Check sheet for the modelled part. Datum: model origin and axes. Units: mm. Round coordinates to 2 decimals unless told otherwise and drop trailing zeros. Loops run counter-clockwise (first coordinate to the right, second up) from the corner with the lowest first, then second, coordinate; pieces in that order, holes last. Notation, with made-up numbers: (-28, 86.25) -> (31, 86.25) arc R17 ccw to (31, 119.25) -> close; hole circle Ø4 at (1.5, 87). An arc over 180 degrees is marked (long way). Use one line per item in the form item = value. Start each with the question number.
(1) Draft check along Z on faces 1 (the cylindrical face through (29.32, 0.01, 86.79)), 2 (the cylindrical face through (-28.289, 0.011, 1.804)), 3 (the cylindrical face through (-24.263, 0.011, 5.805)). Enter one of: released by +Z, released by -Z, zero draft, split by the parting line, or undercut.
(2) Material ranges on probe 1 along X at (y, z) = (-0.2, 24); probe 2 along Z at (x, y) = (2.5, -0.65); probe 3 along X at (y, z) = (0.35, 83), recorded low to high. Write a range as [from, to].
(3) Sectioned sample at B-B (x = -25.75). Record the cut outline in (y, z).
(4) Sectioned sample at A-A (z = 24). Record the cut outline in (x, y), and give its area (3 significant figures).
(5) Go/stop test with flat-tipped pins: pin 1 (0.8 mm diameter, centred on y = 0, z = 87.5, fed in from +X); pin 2 (5 mm diameter, centred on x = -25.75, z = 24, fed in from -Y); pin 3 (0.9 mm diameter, centred on x = -2.6, z = 19, fed in from -Y); pin 4 (0.8 mm diameter, centred on y = 0, z = 85.5, fed in from -X). Record where each tip stops, or that it passes through.
(6) Sectioned sample at C-C (y = 0.05). State how many separate pieces and enclosed holes the cut face has, and give its area (3 significant figures).
from build123d import *

# Parameters (mm, degrees)
SKICA1_W                 = 60
SKICA1_H                 = 95
P_IDAT_VYSUNUT_M1_DEPTH  = 0.8
SKICA3_OUTSIDE_W         = 84.474
SKICA3_OUTSIDE_H         = 119.474
ODEBRAT_VYSUNUT_M2_DEPTH = 100.637141669
SKICA2_W                 = 1.6
SKICA2_H                 = 7.62
ODEBRAT_VYSUNUT_M1_DEPTH = 100.637141669
SKICA4_R                 = 1.5
ODEBRAT_VYSUNUT_M3_DEPTH = 100.637141669
SKICA5_R                 = 1.143
ODEBRAT_VYSUNUT_M4_DEPTH = 100.637141669
SKICA8_R                 = 0.75
ODEBRAT_VYSUNUT_M5_DEPTH = 100.637141669


with BuildPart() as part:
    # Skica1 → Přidat vysunutím1 (new, symmetric)
    with BuildSketch(Plane(origin=(0, 0, 0), x_dir=(1, 0, 0), z_dir=(0, 1, 0))):
        with Locations((0, -47.5)):
            Rectangle(SKICA1_W, SKICA1_H)
    extrude(amount=P_IDAT_VYSUNUT_M1_DEPTH, both=True)

    # Skica3 outside → Odebrat vysunutím2 (cut, through all)
    with BuildSketch(Plane(origin=(0, 0.8, 0), x_dir=(1, 0, 0), z_dir=(0, 1, 0))):
        with Locations((0, -47.5)):
            Rectangle(SKICA3_OUTSIDE_W, SKICA3_OUTSIDE_H)
        with BuildLine():
            Line((-24, 0), (24, 0))
            ThreePointArc((24, 0), (28.242640687, -1.757359313), (30, -6))
            Line((30, -6), (30, -81))
            ThreePointArc((30, -81), (29.302055214, -86.866013328), (27.247191011, -92.404494382))
            ThreePointArc((27.247191011, -92.404494382), (25.488738681, -94.299754206), (23, -95))
            Line((23, -95), (-23, -95))
            ThreePointArc((-23, -95), (-25.488738681, -94.299754206), (-27.247191011, -92.404494382))
            ThreePointArc((-27.247191011, -92.404494382), (-29.302055214, -86.866013328), (-30, -81))
            Line((-30, -81), (-30, -6))
            ThreePointArc((-30, -6), (-28.242640687, -1.757359313), (-24, 0))
        make_face(mode=Mode.SUBTRACT)
    extrude(amount=-ODEBRAT_VYSUNUT_M2_DEPTH, mode=Mode.SUBTRACT)

    # Skica2 → Odebrat vysunutím1 (cut, through all)
    with BuildSketch(Plane(origin=(0, 0.8, 0), x_dir=(1, 0, 0), z_dir=(0, 1, 0))):
        with Locations((-20.8, -86.19)):
            Rectangle(SKICA2_W, SKICA2_H)
        with Locations((20.8, -86.19)):
            Rectangle(SKICA2_W, SKICA2_H)
    extrude(amount=-ODEBRAT_VYSUNUT_M1_DEPTH, mode=Mode.SUBTRACT)

    # Skica4 → Odebrat vysunutím3 (cut, through all)
    with BuildSketch(Plane(origin=(0, 0.8, 0), x_dir=(1, 0, 0), z_dir=(0, 1, 0))):
        with Locations(Location((-25.75, -6, 0), (0, 0, 270))):
            Circle(SKICA4_R)
        with Locations(Location((-25.75, -24, 0), (0, 0, 270))):
            Circle(SKICA4_R)
        with Locations(Location((25.75, -24, 0), (0, 0, 90))):
            Circle(SKICA4_R)
        with Locations(Location((25.75, -6, 0), (0, 0, 90))):
            Circle(SKICA4_R)
    extrude(amount=-ODEBRAT_VYSUNUT_M3_DEPTH, mode=Mode.SUBTRACT)

    # Skica5 → Odebrat vysunutím4 (cut, through all)
    with BuildSketch(Plane.XZ.offset(0.8)):
        with Locations(Location((-7.366, 83, 0), (0, 0, 270))):
            Circle(SKICA5_R)
        with Locations(Location((7.366, 83, 0), (0, 0, 270))):
            Circle(SKICA5_R)
    extrude(amount=-ODEBRAT_VYSUNUT_M4_DEPTH, mode=Mode.SUBTRACT)

    # Skica8 → Odebrat vysunutím5 (cut, through all)
    with BuildSketch(Plane(origin=(0, 0.8, 0), x_dir=(1, 0, 0), z_dir=(0, 1, 0))):
        with Locations(Location((-2.6, -11, 0), (0, 0, 270))):
            Circle(SKICA8_R)
        with Locations(Location((-2.6, -19, 0), (0, 0, 270))):
            Circle(SKICA8_R)
        with Locations(Location((2.6, -19, 0), (0, 0, 90))):
            Circle(SKICA8_R)
        with Locations(Location((2.6, -11, 0), (0, 0, 90))):
            Circle(SKICA8_R)
    extrude(amount=-ODEBRAT_VYSUNUT_M5_DEPTH, mode=Mode.SUBTRACT)


solid = part.part
Checks:
q1.face_1 = released by +Z
q1.face_2 = released by -Z
q1.face_3 = undercut
q2.probe_1 = [-30, -27.25], [-24.25, 24.25], [27.25, 30]
q2.probe_2 = [0, 10.26], [11.74, 18.26], [19.74, 95]
q2.probe_3 = [-29.92, -21.6], [-20, -8.51], [-6.22, 6.22], [8.51, 20], [21.6, 29.92]
q3.outline = (-0.8, 0.26) -> (0.8, 0.26) -> (0.8, 4.5) -> (-0.8, 4.5) -> close; (-0.8, 7.5) -> (0.8, 7.5) -> (0.8, 22.5) -> (-0.8, 22.5) -> close; (-0.8, 25.5) -> (0.8, 25.5) -> (0.8, 94.13) -> (-0.8, 94.13) -> close
q4.outline = (-30, -0.8) -> (-27.25, -0.8) -> (-27.25, 0.8) -> (-30, 0.8) -> close; (-24.25, -0.8) -> (24.25, -0.8) -> (24.25, 0.8) -> (-24.25, 0.8) -> close; (27.25, -0.8) -> (30, -0.8) -> (30, 0.8) -> (27.25, 0.8) -> close
q4.area = 86.4 mm2
q5.pin_1 = 29.24
q5.pin_2 = -0.8
q5.pin_3 = through
q5.pin_4 = -29.66
q6.separate_pieces = 1
q6.enclosed_holes = 12
q6.area = 5,580 mm2
